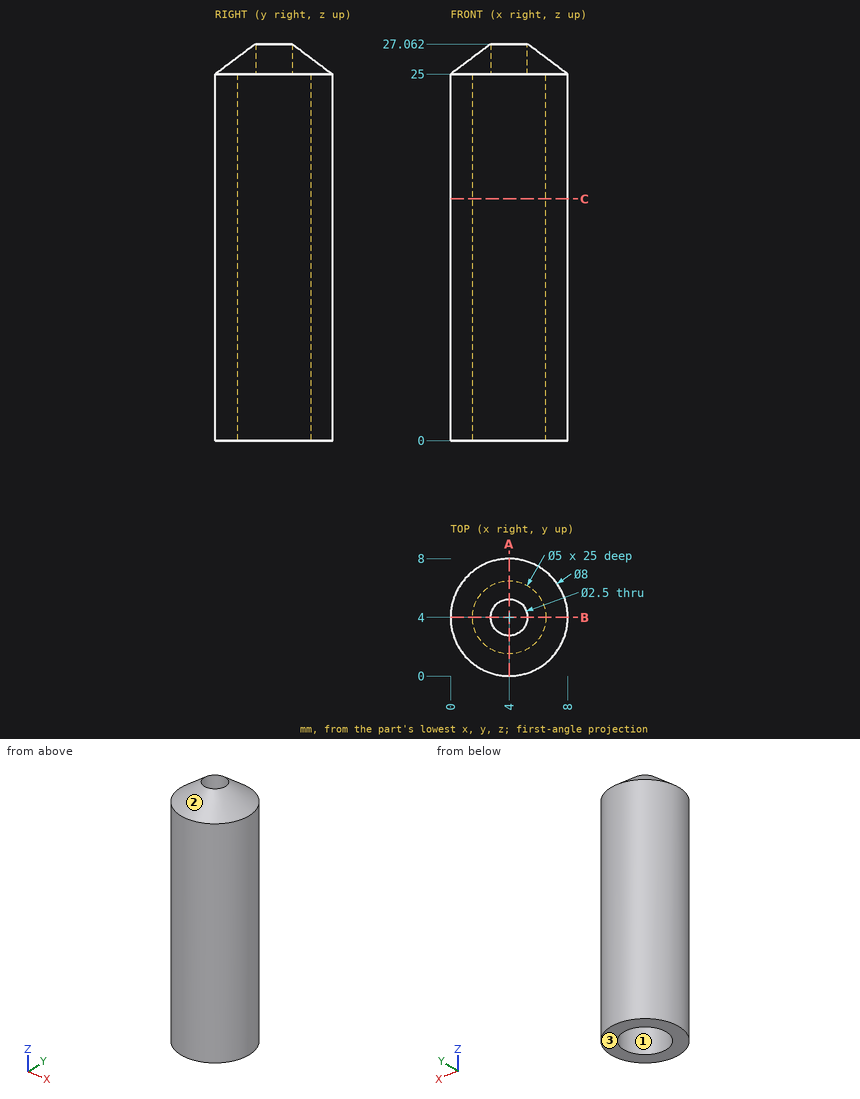
Job drawing, mm, ordinate dimensions from the low corner. One solid piece. Coordinates: 2 decimals unless noted, no trailing zeros. Write each loop counter-clockwise with the first axis right and the second up, starting at its lowest first coordinate (ties: lowest second). Pieces come first, ordered by that corner, then holes. Notation, with made-up numbers: M 77,-10.75 L 118,-10.75 A21 cw 118,24.25 Z; hole C 68.5,46.5 d9. An arc over 180 degrees is marked long. Answer as a JSON object with one key per item and string values. Group by question number.
1) Pin check, flat tips, straight feed: pin 1 Ø3 at (x, z) = (2, 8) entering from -Y; pin 2 Ø1 at (y, z) = (7, 8.5) entering from -X. Stop position of each tip, or through.
2) Wall check: line 1 (Y direction, x = 4, z = 17.5); line 2 (Y direction, x = 6.25, z = 24.25) (1 decimal). Give the ranges that are in metal, low to high. Write a range as from..to.
3) Saw through at C-C (z = 16.5). Write the cut outline in (x, y).
4) Saw through at A-A (x = 4). Write the cut outline in (y, z).
5) Mould opens along Y. For the marked faces 1, 2 and 3 say: +Y half, -Y half, draft (parallel to the pull), parting line (faces both ways), or undercut.
Values follow:
{
 "1": {"pin 1": "stops at y = 0.03", "pin 2": "stops at x = 0.88"},
 "2": {"line 1": "y = 0..1.5, 6.5..8", "line 2": "y = 0.7..2.9, 5.1..7.3"},
 "3": {"outline": "C 4,4 d8; hole C 4,4 d5"},
 "4": {"outline": "M 0,0 L 1.5,0 L 1.5,25 L 2.75,25 L 2.75,27.06 L 0,25 Z; M 5.25,25 L 6.5,25 L 6.5,0 L 8,0 L 8,25 L 5.25,27.06 Z"},
 "5": {"face 1": "undercut", "face 2": "parting line", "face 3": "draft"}
}
